from build123d import *

# Parameters (mm, degrees)
F0_W     = 23
F0_H     = 28
F1_DEPTH = 30
F2_R     = 2
F3_R     = 2
F4_R     = 2
F5_R     = 2
F6_R     = 2
F7_T     = 2
F8_R     = 2


# Not quite as in the source:
# - a feature of the source that left no trace in its solid (it failed there, or was rolled back) is left out
# - a shell that OpenCascade refuses in one call is made with other operations: the cavity is built on its own and cut out


with BuildPart() as f1:
    # F0 (on Top) → F1 (new body)
    with BuildSketch(Plane.XY):
        with Locations((-41.8064879576, 45.8027429283)):
            Rectangle(F0_W, F0_H)
    extrude(amount=F1_DEPTH)

    # F2
    f2_edges = [f1.edges().sort_by_distance(p)[0] for p in [
        (-30.306488, 31.802743, 15),
    ]]
    fillet(f2_edges, radius=F2_R)

    # F3
    f3_edges = [f1.edges().sort_by_distance(p)[0] for p in [
        (-30.306488, 59.802743, 15),
    ]]
    fillet(f3_edges, radius=F3_R)

    # F4
    f4_edges = [f1.edges().sort_by_distance(p)[0] for p in [
        (-53.306488, 31.802743, 15),
    ]]
    fillet(f4_edges, radius=F4_R)

    # F5
    f5_edges = [f1.edges().sort_by_distance(p)[0] for p in [
        (-53.306488, 59.802743, 15),
    ]]
    fillet(f5_edges, radius=F5_R)

    # F6
    f6_edges = [f1.edges().sort_by_distance(p)[0] for p in [
        (-41.806488, 31.802743, 30),
    ]]
    fillet(f6_edges, radius=F6_R)

    # F7: shell of thickness 2, made by hand


with BuildPart() as f7_core1:
    # F7_t2: copy of F1
    add(f1.part)

    # the walls: a layer under each face that stays
    f7_faces = [f7_core1.faces().sort_by_distance(p)[0] for p in [
        (-53.3064879576, 45.8027429283, 14),
        (-41.8064879576, 59.8027429283, 14),
        (-41.8064879576, 45.8027429283, 30),
        (-41.8064879576, 31.8027429283, 14),
        (-30.3064879576, 45.8027429283, 14),
    ]]
    thicken(f7_faces, amount=-F7_T, mode=Mode.SUBTRACT)


with BuildPart() as f1_1:
    add(f1.part)

    # what is left inside the walls is the cavity
    f7_cavity = [f7_core1.part.solids().sort_by_distance(p)[0] for p in [
        (-51.286488, 45.802743, 18.666667),
    ]]
    add(f7_cavity, mode=Mode.SUBTRACT)

    # F8
    f8_edges = [f1_1.edges().sort_by_distance(p)[0] for p in [
        (-51.306488, 57.802743, 14),
        (-51.306488, 33.802743, 14),
        (-32.306488, 33.802743, 14),
        (-32.306488, 57.802743, 14),
    ]]
    fillet(f8_edges, radius=F8_R)


solid = f1_1.part
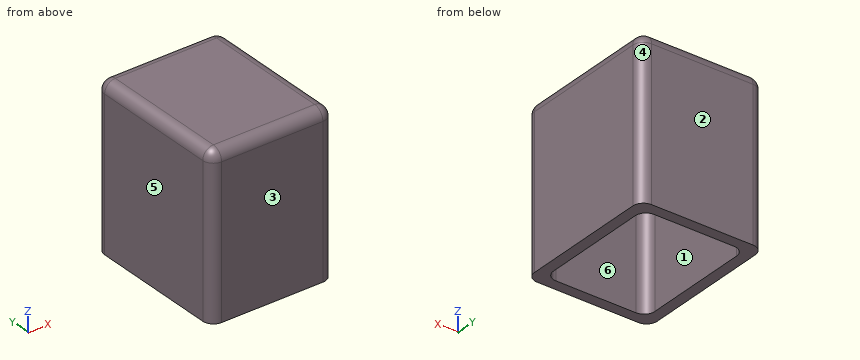
Geometry check sheet. Reference: the model listing, model coordinates, mm. Face numbers are marked on the shaded views. A direction names the side the tool comes from. Give positions to 0.01 mm unless a question says otherwise; leave off trailing zeros. Loops run counter-clockwise (first coordinate to the right, second up) from the corner with the lowest first, then second, coordinate; pieces in that order, holes last. Notation, with made-up numbers: M 74.25,45.5 L 89.25,45.5 A26 ccw 89.25,79.5 Z; hole C 21.5,-0.75 d5. An arc over 180 degrees is marked long. Write each question's results on one line, items separated by ' | '.
1) Section check B-B, the plane x = -46. Record the boundary of the cut face in (y, z).
Answers follow:
outline: M 31.8,0 L 33.8,0 L 33.8,28 L 57.8,28 L 57.8,0 L 59.8,0 L 59.8,28 A2 ccw 57.8,30 L 33.8,30 A2 ccw 31.8,28 Z
2) Tool access check on the marked faces 1 and 2. Record the directions out of +Z, -Z, +X, -X, +Y, -Y that give a thin tool (end or side, any length) a straight path to the whole face; none if there is none.
Answers follow:
face 1: -Z | face 2: +Z, -Z, +X, -X, +Y
3) Section check C-C, the plane y = 39.5. Record the boundary of the cut face in (x, z), plus the area to 3 significant figures.
Answers follow:
outline: M -53.31,0 L -51.31,0 L -51.31,28 L -32.31,28 L -32.31,0 L -30.31,0 L -30.31,28 A2 ccw -32.31,30 L -51.31,30 A2 ccw -53.31,28 Z | area: 156 mm2
4) Thickness scan on line 1 (Y direction, x = -40.75, z = 21.25); line 2 (X direction, y = 53, z = 24.25); line 3 (Z direction, x = -41.75, y = 55.5). Record the ranges inside material, lowest first.
Answers follow:
line 1: 31.8 to 33.8, 57.8 to 59.8 | line 2: -53.31 to -51.31, -32.31 to -30.31 | line 3: 28 to 30
5) Section check A-A, the plane z = 9. Record the boundary of the cut face in (x, y), plus the area to 3 significant figures.
Answers follow:
outline: M -53.31,33.8 A2 ccw -51.31,31.8 L -32.31,31.8 A2 ccw -30.31,33.8 L -30.31,57.8 A2 ccw -32.31,59.8 L -51.31,59.8 A2 ccw -53.31,57.8 Z; hole M -51.31,35.8 A2 ccw -49.31,33.8 L -34.31,33.8 A2 ccw -32.31,35.8 L -32.31,55.8 A2 ccw -34.31,57.8 L -49.31,57.8 A2 ccw -51.31,55.8 Z | area: 188 mm2
6) Gauge pin test, flat end, axial feed: pin 1 (1.5 mm diameter, centred on x = -48, y = 57, fed in from -Z). Record the tip position at first contact, or that the pin passes through.
Answers follow:
pin 1: z = 28
7) Release check for a two-part mould opening along Y. For the marked faces 3, 4, 5 and 6 record: +Y half, -Y half, draft (parallel to the pull), parting line (faces both ways), or undercut.
Answers follow:
face 3: -Y half | face 4: +Y half | face 5: draft | face 6: undercut
